Can you work these out from the model? Positions are in its coordinate system, mm. A direction names the side the tool comes from. Give positions to 0.01 mm unless a question says otherwise; leave off trailing zeros. Order: outer loops, then holes, each group sorted by start corner. A loop starts at its lowest first (then second) coordinate and runs counter-clockwise, first axis right, second up. Notation, with made-up numbers: M 71,87.5 L 92,87.5 A32 ccw 92,119.5 Z; hole C -26,18.25 d8. An arc over 180 degrees is marked long. Write each question's results on one line, items separated by ' | '.
from build123d import *

# Parameters (mm, degrees)
BOSS_EXTRUDE1_DEPTH = 10
SKETCH2_R           = 2.85
CUT_EXTRUDE1_DEPTH  = 14
SKETCH5_R           = 5
CUT_EXTRUDE2_DEPTH  = 5.5
BOSS_EXTRUDE3_DEPTH = 10
SKETCH8_W           = 195
SKETCH8_H           = 5.03
BOSS_EXTRUDE4_DEPTH = 7.5
BOSS_EXTRUDE5_START = -5.03
BOSS_EXTRUDE5_DEPTH = 6.5
CUT_EXTRUDE3_DEPTH  = 17.06
SKETCH10_W          = 195
SKETCH10_H          = 7
CUT_EXTRUDE4_DEPTH  = 5
SKETCH11_R          = 3.175
CUT_EXTRUDE5_DEPTH  = 23
SKETCH12_R          = 7.5
CUT_EXTRUDE6_DEPTH  = 1.47
SKETCH14_W          = 7.794228634
SKETCH14_H          = 5.03
BOSS_EXTRUDE6_DEPTH = 1.5
CUT_EXTRUDE7_DEPTH  = 4.5
BOSS_EXTRUDE7_DEPTH = 5.03
LPATTERN4_COUNT     = 5
LPATTERN4_PITCH     = 25
CHAMFER1_SIZE       = 1
CHAMFER2_SIZE       = 1


with BuildPart() as part:
    # Sketch1 → Boss-Extrude1 (new body)
    with BuildSketch(Plane(origin=(0, 0, 0), x_dir=(1, 0, 0), z_dir=(0, 1, 0))):
        Polygon((48.707649013, 0), (34.441508913, 34.441508913), (0, 48.707649013), (-34.441508913, 34.441508913), (-48.707649013, 0), (-34.441508913, -34.441508913), (0, -48.707649013), (34.441508913, -34.441508913), align=None)
    extrude(amount=-BOSS_EXTRUDE1_DEPTH)

    # Sketch2 → Cut-Extrude1 (cut)
    with BuildSketch(Plane(origin=(0, 0, 0), x_dir=(1, 0, 0), z_dir=(0, 1, 0))):
        with Locations((-35.355339059, 0)):
            Circle(SKETCH2_R)
        with Locations((-25, 25)):
            Circle(SKETCH2_R)
        with Locations((0, 35.355339059)):
            Circle(SKETCH2_R)
        with Locations((25, 25)):
            Circle(SKETCH2_R)
        with Locations((25, -25)):
            Circle(SKETCH2_R)
        with Locations((0, -35.355339059)):
            Circle(SKETCH2_R)
        with Locations((-25, -25)):
            Circle(SKETCH2_R)
    extrude(amount=-CUT_EXTRUDE1_DEPTH, mode=Mode.SUBTRACT)

    # Sketch5 → Cut-Extrude2 (cut)
    with BuildSketch(Plane(origin=(0, 0, 0), x_dir=(1, 0, 0), z_dir=(0, 1, 0))):
        with Locations((-35.355339059, 0)):
            Circle(SKETCH5_R)
        with Locations((-25, 25)):
            Circle(SKETCH5_R)
        with Locations((0, 35.355339059)):
            Circle(SKETCH5_R)
        with Locations((25, 25)):
            Circle(SKETCH5_R)
        with Locations((25, -25)):
            Circle(SKETCH5_R)
        with Locations((0, -35.355339059)):
            Circle(SKETCH5_R)
        with Locations((-25, -25)):
            Circle(SKETCH5_R)
    extrude(amount=-CUT_EXTRUDE2_DEPTH, mode=Mode.SUBTRACT)

    # Sketch7 → Boss-Extrude3 (add)
    with BuildSketch(Plane(origin=(0, 0, 0), x_dir=(1, 0, 0), z_dir=(0, 1, 0))):
        Polygon((45, -10), (34.441508913, -34.441508913), (34.441508913, 34.441508913), (45, 10), (195, 10), (195, -10), align=None)
    extrude(amount=-BOSS_EXTRUDE3_DEPTH)

    # Sketch8 → Boss-Extrude4 (add)
    with BuildSketch(Plane(origin=(0, 0, 0), x_dir=(1, 0, 0), z_dir=(0, 1, 0))):
        with Locations((97.5, -6.015)):
            Rectangle(SKETCH8_W, SKETCH8_H)
        with Locations((97.5, 6.015)):
            Rectangle(SKETCH8_W, SKETCH8_H)
    extrude(amount=BOSS_EXTRUDE4_DEPTH)

    # Sketch13 → Boss-Extrude5 (add)
    with BuildSketch(Plane(origin=(0, 0, -8.53), x_dir=(-1, 0, 0), z_dir=(0, 0, -1)).offset(BOSS_EXTRUDE5_START)):
        Polygon((-166.339745962, 3.75), (-170.669872981, 11.25), (-179.330127019, 11.25), (-183.660254038, 3.75), (-183.660254038, -3.75), (-166.339745962, -3.75), align=None)
        Polygon((-168.937822174, 3.75), (-171.968911087, 9), (-178.031088913, 9), (-181.062177826, 3.75), (-178.031088913, -1.5), (-171.968911087, -1.5), align=None, mode=Mode.SUBTRACT)
    boss_extrude5 = extrude(amount=BOSS_EXTRUDE5_DEPTH)

    # Sketch9 → Cut-Extrude3 (cut)
    with BuildSketch(Plane.XY.offset(8.53)):
        Polygon((0, 0), (12.990381057, 7.5), (0, 7.5), align=None)
        Polygon((182.009618943, 7.5), (195, 0), (195, 7.5), align=None)
    extrude(amount=-CUT_EXTRUDE3_DEPTH, mode=Mode.SUBTRACT)

    # Sketch10 → Cut-Extrude4 (cut)
    with BuildSketch(Plane(origin=(0, 0, 0), x_dir=(1, 0, 0), z_dir=(0, 1, 0))):
        with Locations((97.5, 0)):
            Rectangle(SKETCH10_W, SKETCH10_H)
    extrude(amount=-CUT_EXTRUDE4_DEPTH, mode=Mode.SUBTRACT)

    # Sketch11 → Cut-Extrude5 (cut)
    with BuildSketch(Plane.XY.offset(8.53)):
        with Locations((175, 3.75)):
            Circle(SKETCH11_R)
    cut_extrude5 = extrude(amount=-CUT_EXTRUDE5_DEPTH, mode=Mode.SUBTRACT)

    # Sketch12 → Cut-Extrude6 (cut)
    with BuildSketch(Plane.XY.offset(10)):
        with Locations((175, 3.75)):
            Circle(SKETCH12_R)
    cut_extrude6 = extrude(amount=-CUT_EXTRUDE6_DEPTH, mode=Mode.SUBTRACT)

    # Sketch14 → Boss-Extrude6 (add)
    with BuildSketch(Plane(origin=(0, 7.5, 0), x_dir=(1, 0, 0), z_dir=(0, 1, 0))):
        with Locations((175, 6.015)):
            Rectangle(SKETCH14_W, SKETCH14_H)
    boss_extrude6 = extrude(amount=BOSS_EXTRUDE6_DEPTH)

    # Sketch15 → Cut-Extrude7 (cut)
    with BuildSketch(Plane(origin=(0, 0, -10), x_dir=(-1, 0, 0), z_dir=(0, 0, -1))):
        Polygon((-168.937822174, 3.75), (-171.968911087, 9), (-178.031088913, 9), (-181.062177826, 3.75), (-178.031088913, -1.5), (-171.968911087, -1.5), align=None)
    cut_extrude7 = extrude(amount=-CUT_EXTRUDE7_DEPTH, mode=Mode.SUBTRACT)

    # Sketch16 → Boss-Extrude7 (add)
    with BuildSketch(Plane.XY.offset(8.53)):
        Polygon((168.504809472, 7.5), (170.669872981, 11.25), (179.330127019, 11.25), (181.495190528, 7.5), align=None)
    boss_extrude7 = extrude(amount=-BOSS_EXTRUDE7_DEPTH)

    # LPattern4: Boss-Extrude5, Cut-Extrude5, Cut-Extrude6, Boss-Extrude6, Cut-Extrude7, Boss-Extrude7 ×5
    with Locations(*[(-i * LPATTERN4_PITCH, 0, 0) for i in range(1, LPATTERN4_COUNT)]):
        add(boss_extrude5)
        add(cut_extrude5, mode=Mode.SUBTRACT)
        add(cut_extrude6, mode=Mode.SUBTRACT)
        add(boss_extrude6)
        add(cut_extrude7, mode=Mode.SUBTRACT)
        add(boss_extrude7)

    # Chamfer1
    chamfer1_edges = [part.edges().sort_by_distance(p)[0] for p in [
        (-40.355339059, 0, 0),
        (-30, 0, 25),
        (-5, 0, 35.355339059),
        (20, 0, 25),
        (20, 0, -25),
        (-5, 0, -35.355339059),
        (-30, 0, -25),
    ]]
    chamfer(chamfer1_edges, length=CHAMFER1_SIZE)

    # Chamfer2
    chamfer2_edges = [part.edges().sort_by_distance(p)[0] for p in [
        (162.5, 7.5, -8.53),
        (40.747595264, 7.5, -3.5),
        (6.495190528, 3.75, -3.5),
        (40.747595264, 7.5, 8.53),
        (6.495190528, 3.75, 3.5),
        (6.495190528, 3.75, 8.53),
        (6.495190528, 3.75, -8.53),
        (162.5, 7.5, 3.5),
        (162.5, 7.5, -3.5),
        (137.5, 7.5, -8.53),
        (137.5, 7.5, -3.5),
        (112.5, 7.5, -8.53),
        (112.5, 7.5, -3.5),
        (87.5, 7.5, -8.53),
        (87.5, 7.5, -3.5),
        (40.747595264, 7.5, -8.53),
        (137.5, 7.5, 3.5),
        (162.5, 7.5, 8.53),
        (112.5, 7.5, 3.5),
        (137.5, 7.5, 8.53),
        (87.5, 7.5, 3.5),
        (112.5, 7.5, 8.53),
        (40.747595264, 7.5, 3.5),
        (87.5, 7.5, 8.53),
    ]]
    chamfer(chamfer2_edges, length=CHAMFER2_SIZE)


solid = part.part
(1) I need wall thicknesses on L1, parallel to Z at x = 0, y = -7.15; L2, parallel to Z at x = 118.5, y = 3.5; L3, parallel to Z at x = 4, y = -4. Which ranges of each line are inside material? Lowest first, please. Write a range as from..to.
Data:
L1: z = -48.71..-38.21, -32.51..32.51, 38.21..48.71 | L2: z = -10..-3.5, 3.5..8.53 | L3: z = -47.05..-38.36, -32.36..-3.5, 3.5..32.36, 38.36..47.05
(2) We'd pull the mould along Y, two halves only. Please class faces 6 (the face through (175, 9, -8)), 7 (the face through (94.6, 9.4, 6.1)), 8 (the face through (188, 3, -8.53)): +Y half, -Y half, draft (parallel to the pull), parting line (faces both ways), or undercut.
Data:
face 6: undercut | face 7: +Y half | face 8: draft
(3) For faces 1 (the face through (96, -5, 0)), 2 (the face through (-23.685, -7.719, 27.528)), 3 (the face through (6.658, 3.258, -8.037)), 4 (the face through (150, -1.5, -8)), 5 (the face through (2, -5.5, 38)), which set-ups out of +Z, -Z, +X, -X, +Y, -Y let a thin tool reach every point of the face, with its end or its side?
Data:
face 1: +X, +Y | face 2: +Y, -Y | face 3: -Z, -X, +Y | face 4: -Z | face 5: +Y
(4) Imagine slicing it at B-B, the plane x = -25. Write out the boundary of the cut face in (y, z), plus the area to 3 significant figures.
Data:
outline: M -10,-38.35 L 0,-38.35 L 0,-31 L -1,-30 L -5.5,-30 L -5.5,-27.85 L -10,-27.85 Z; M -10,-22.15 L -5.5,-22.15 L -5.5,-20 L -1,-20 L 0,-19 L 0,19 L -1,20 L -5.5,20 L -5.5,22.15 L -10,22.15 Z; M -10,27.85 L -5.5,27.85 L -5.5,30 L -1,30 L 0,31 L 0,38.35 L -10,38.35 Z | area: 604 mm2
(5) Will these pins go through, and if not, where does the flat tip stop? P1, Ø10, axis at x = 5.5, y = 0, coming from the -Z side; P2, Ø10, axis at x = 61.5, z = -0.5, coming from the +Y side; P3, Ø4, axis at x = 6.5, y = 5.5, coming from the -Z side; P4, Ø5, axis at x = 75, y = 3.75, coming from the +Z side (1 decimal).
Data:
P1: stops at z = -48.5 | P2: stops at y = 7.5 | P3: stops at z = -8.02 | P4: passes through
(6) Imagine slicing it at A-A, the plane x = 100. Write out the boundary of the cut face in (y, z) (3 decimals).
Data:
outline: M -10,-10 L -1.5,-10 L -1.5,-5.5 L 0.575,-5.5 L 0.575,-3.5 L -5,-3.5 L -5,3.5 L 0.575,3.5 L 0.575,8.53 L -3.75,8.53 L -3.75,10 L -10,10 Z; M 6.925,-5.5 L 9,-5.5 L 9,-10 L 11.25,-10 L 11.25,-3.5 L 6.925,-3.5 Z; M 6.925,3.5 L 11.25,3.5 L 11.25,8.53 L 6.925,8.53 Z
